from build123d import *

# Parameters (mm, degrees)
F1_DEPTH = 57.15
F3_D     = 12.7


# Not quite as in the source:
# - a length typed as a fraction of an inch, garbled in the dataset ("3 / 203.2 mm" for 3/8 in), is restored


with BuildPart() as f1:
    # F0 (on Front) → F1 (new body, symmetric)
    with BuildSketch(Plane.XZ):
        Polygon((-627.0625, 4.7625), (-660.4, 4.7625), (-660.4, 0), (-622.3, 0), (-622.3, 203.2), (622.3, 203.2), (622.3, 0), (660.4, 0), (660.4, 4.7625), (627.0625, 4.7625), (627.0625, 207.9625), (-627.0625, 207.9625), align=None)
    extrude(amount=F1_DEPTH, both=True)

    # F3 (through all)
    with Locations(Plane.XY.offset(4.7625)):
        with Locations((-642.9375, 38.1), (-642.9375, -38.1), (642.9375, 38.1), (642.9375, -38.1)):
            Hole(F3_D / 2)


solid = f1.part
Geometry check sheet. Reference: the model listing, model coordinates, mm. A direction names the side the tool comes from. Give positions to 0.01 mm unless a question says otherwise; leave off trailing zeros. Order: outer loops, then holes, each group sorted by start corner. A loop starts at its lowest first (then second) coordinate and runs counter-clockwise, first axis right, second up.
1) Draft check along X on faces 1 (the flat face through (-9, -1, 203.2)), 2 (the flat face through (627.062, -1, 105)), 3 (the flat face through (-3, -57.15, 205)). Enter one of: released by +X, released by -X, zero draft, split by the parting line, or undercut.
Results are:
face 1: undercut
face 2: released by +X
face 3: zero draft
2) Gauge pin test, flat ends, axial feed: pin 1 (20.5 mm diameter, centred on x = -642.94, y = 38.1, fed in from -Z); pin 2 (10 mm diameter, centred on x = -86.5, y = 7, fed in from -Z); pin 3 (1 mm diameter, centred on y = 41, z = 96.5, fed in from -X); pin 4 (5 mm diameter, centred on y = 12, z = 172.5, fed in from +X). Record the tip position at first contact, or that the pin passes through.
Results are:
pin 1: stops at z = 0
pin 2: stops at z = 203.2
pin 3: stops at x = -627.06
pin 4: stops at x = 627.06
3) Cross-section at B-B (y = 0.5). Record the boundary of the cut face in (x, z), then the cut area to 3 significant figures.
Results are:
outline: (-660.4, 0) - (-622.3, 0) - (-622.3, 203.2) - (622.3, 203.2) - (622.3, 0) - (660.4, 0) - (660.4, 4.76) - (627.06, 4.76) - (627.06, 207.96) - (-627.06, 207.96) - (-627.06, 4.76) - (-660.4, 4.76) - close
area: 8,230 mm2
4) Cross-section at C-C (x = -350). Record the boundary of the cut face in (y, z).
Results are:
outline: (-57.15, 203.2) - (57.15, 203.2) - (57.15, 207.96) - (-57.15, 207.96) - close
5) Tool access check on faces 4 (the flat face through (-627.062, -1, 108)), 5 (the flat face through (644, -1, 4.762)), 6 (the flat face through (-622.3, -1, 100)), 7 (the flat face through (-642, -1, 0)), 8 (the flat face through (-3, 57.15, 205)). Record the directions out of +Z, -Z, +X, -X, +Y, -Y that give a thin tool (end or side, any length) a straight path to the whole face; none if there is none.
Results are:
face 4: +Z, -X, +Y, -Y
face 5: +Z, +X, +Y, -Y
face 6: -Z, +Y, -Y
face 7: -Z, +X, -X, +Y, -Y
face 8: +Z, -Z, +X, -X, +Y
6) Cross-section at A-A (z = 129). Record the boundary of the cut face in (x, y).
Results are:
outline: (-627.06, -57.15) - (-622.3, -57.15) - (-622.3, 57.15) - (-627.06, 57.15) - close; (622.3, -57.15) - (627.06, -57.15) - (627.06, 57.15) - (622.3, 57.15) - close
7) Material ranges on probe 1 along X at (y, z) = (-38, 1); probe 2 along X at (y, z) = (29, 105); probe 3 along Z at (x, y) = (590, 12.5), recorded low to high.
Results are:
probe 1: x = -660.4 to -649.29, -636.59 to -622.3, 622.3 to 636.59, 649.29 to 660.4
probe 2: x = -627.06 to -622.3, 622.3 to 627.06
probe 3: z = 203.2 to 207.96
